Could you check a few things on this drawing? It's one solid part, dimensions in mm from its lowest x, y, z. A direction names the side the tool comes from. Give positions to 0.01 mm unless a question says otherwise; leave off trailing zeros. Order: outer loops, then holes, each group sorted by start corner. A loop starts at its lowest first (then second) coordinate and runs counter-clockwise, first axis right, second up.
Item 1: I want a section at A-A, the plane x = 14. Write out the boundary of the cut face in (y, z).
Item 2: If I drill on line 1 along X through (y, z) = (11, 125); line 2 along Z through (x, y) = (49, 110.5) (1 decimal); line 3 along Y through (x, z) = (29, 221) (1 decimal), over which ranges is the centre line in solid material (lowest first)?
Item 3: I'm going to push flat-ended pins straight in: pin 1 Ø3 at (x, y) = (26, 108.5) entering from +Z (1 decimal); pin 2 Ø6 at (x, y) = (37.5, 89.5) entering from -Z (1 decimal); pin 3 Ø1 at (x, y) = (85.5, 59.5) entering from -Z (1 decimal); pin 4 Ø8 at (y, z) = (108, 215.5) entering from +X. Where does each tip first touch, or does it pass through?
Item 4: I want a section at C-C, the plane z = 93.5. Write out the boundary of the cut face in (x, y), then the cut area to 3 significant figures.
Item 5: I want a section at B-B, the plane y = 29. Write out the boundary of the cut face in (x, z) (1 decimal).
Item 6: Which directions (+Z, -Z, +X, -X, +Y, -Y) give clear straight access to the entire face, cutting with the end or side of a thin tool? Please do the marked faces 1 and 2.
Item 7: I want a section at D-D, the plane y = 84. Write out the boundary of the cut face in (x, z), then the cut area to 3 significant figures.
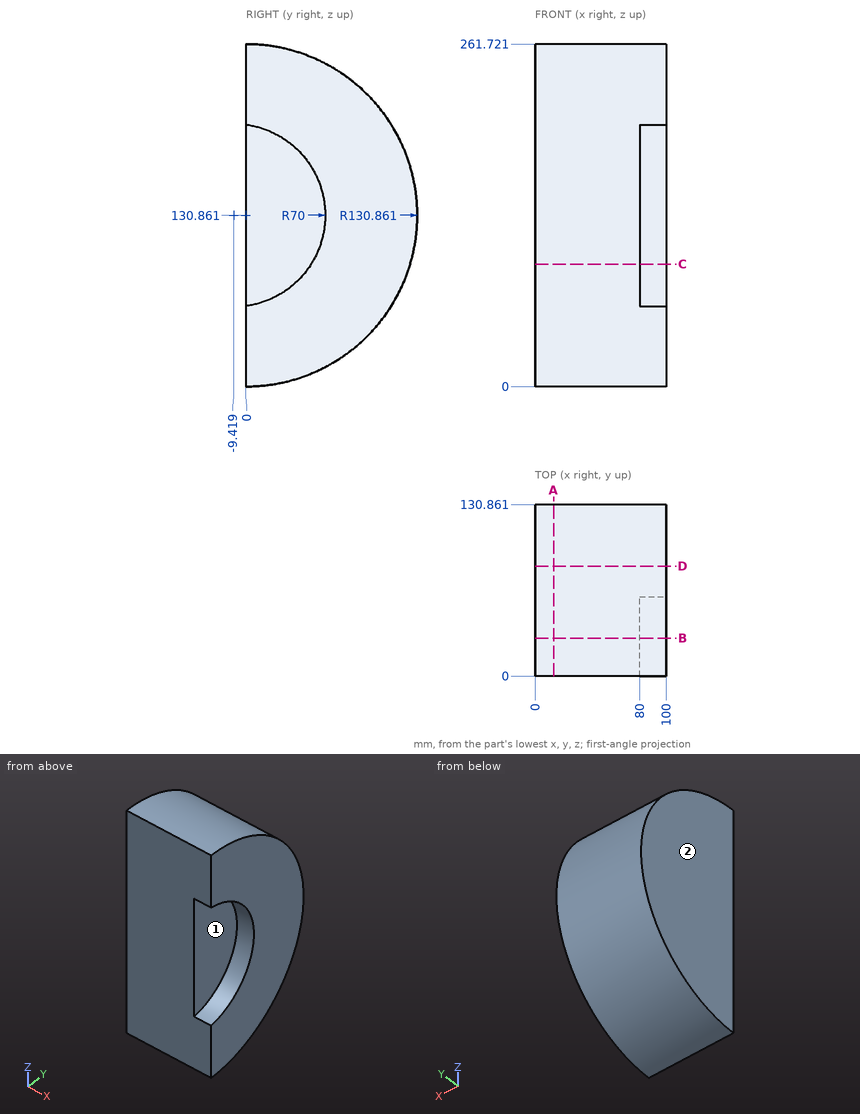
Results list:
1. outline: (0, 0) arc R130.86 ccw to (0, 261.72) - close
2. line 1: x = 0 to 80
2. line 2: z = 60.8 to 201
2. line 3: y = 0 to 94.9
3. pin 1: stops at z = 206.2
3. pin 2: stops at z = 32.7
3. pin 3: stops at z = 14.1
3. pin 4: passes through
4. outline: (0, 0) - (80, 0) - (80, 49.78) - (100, 49.78) - (100, 125.41) - (0, 125.41) - close
4. area: 11,500 mm2
5. outline: (0, 3.3) - (100, 3.3) - (100, 72.3) - (80, 72.3) - (80, 189.4) - (100, 189.4) - (100, 258.5) - (0, 258.5) - close
6. face 1: +X, -Y
6. face 2: +Z, -Z, -X, +Y, -Y
7. outline: (0, 30.52) - (100, 30.52) - (100, 231.2) - (0, 231.2) - close
7. area: 20,100 mm2
